CAD build for the part. Positions are in the model's coordinates, mm. Coordinates: 2 decimals unless noted, no trailing zeros. Order: outer loops, then holes, each group sorted by start corner. A loop starts at its lowest first (then second) coordinate and runs counter-clockwise, first axis right, second up. Notation, with made-up numbers: M 6,4 L 15,4 A26 ccw 15,30 Z; hole C 75.5,-21 d8. An arc over 180 degrees is marked long. One line per item, written item: value.
from build123d import *

# Parameters (mm, degrees)
SKETCH_1_R      = 1.35
EXTRUDE_1_DEPTH = 3
CHAMFER_1_SIZE  = 0.6
CHAMFER_2_SIZE  = 0.2


with BuildPart() as part:
    # ｽｹｯﾁ1 → ﾎﾞｽ - 押し出し1 (new body)
    with BuildSketch(Plane.XY):
        Polygon((3.175426481, 0), (1.58771324, 2.75), (-1.58771324, 2.75), (-3.175426481, 0), (-1.58771324, -2.75), (1.58771324, -2.75), align=None)
        Circle(SKETCH_1_R, mode=Mode.SUBTRACT)
    extrude(amount=EXTRUDE_1_DEPTH)

    # 面取り1
    chamfer_1_edges = [part.edges().sort_by_distance(p)[0] for p in [
        (0, 2.75, 3),
        (-2.38156986, 1.375, 3),
        (-2.38156986, -1.375, 3),
        (0, -2.75, 3),
        (2.38156986, -1.375, 3),
        (2.38156986, 1.375, 3),
    ]]
    chamfer(chamfer_1_edges, length=CHAMFER_1_SIZE)

    # 面取り2
    chamfer_2_edges = [part.edges().sort_by_distance(p)[0] for p in [
        (-1.35, 0, 0),
        (-1.35, 0, 3),
    ]]
    chamfer(chamfer_2_edges, length=CHAMFER_2_SIZE)


solid = part.part
Q1. Mould opens along X. For faces 1 (the face through (-0.29, -1.32, 1.48)), 2 (the face through (2, 0, 3)), 3 (the face through (-2.37, 1.394, 1.183)) say: released by +X, released by -X, zero draft, split by the parting line, or undercut.
Recorded:
face 1: undercut
face 2: zero draft
face 3: released by -X
Q2. Drill centre lines: line 1 along Y through (x, z) = (0, 2.2); line 2 along Y through (x, z) = (1, 2.45); line 3 along X through (y, z) = (0.6, 2.6). Where is each one in solid material? Low to high.
Recorded:
line 1: y = -2.75 to -1.35, 1.35 to 2.75
line 2: y = -2.7 to -0.91, 0.91 to 2.7
line 3: x = -2.6 to -1.21, 1.21 to 2.6
Q3. Slice it at D-D (x = 2.25). List the corners of the cut face in (y, z).
Recorded:
outline: M -1.6,0 L 1.6,0 L 1.6,2.4 L 0.4,3 L -0.4,3 L -1.6,2.4 Z
Q4. Slice it at A-A (z = 0.95). List the corners of the cut face in (x, y).
Recorded:
outline: M -3.18,0 L -1.59,-2.75 L 1.59,-2.75 L 3.18,0 L 1.59,2.75 L -1.59,2.75 Z; hole C 0,0 d2.7
Q5. Slice it at C-C (y = 1.95). List the corners of the cut face in (x, z).
Recorded:
outline: M -2.05,0 L 2.05,0 L 2.05,2.4 L 1.36,3 L -1.36,3 L -2.05,2.4 Z
Q6. Pin check, flat tip, straight feed: pin 1 Ø3 at (x, y) = (2, -0.5) entering from -Z. Stop position of the tip, or through.
Recorded:
pin 1: stops at z = 0
Q7. Slice it at B-B (x = 0). List the corners of the cut face in (y, z).
Recorded:
outline: M -2.75,0 L -1.55,0 L -1.35,0.2 L -1.35,2.8 L -1.55,3 L -2.15,3 L -2.75,2.4 Z; M 1.35,0.2 L 1.55,0 L 2.75,0 L 2.75,2.4 L 2.15,3 L 1.55,3 L 1.35,2.8 Z
